```python
from build123d import *

# Parameters (mm, degrees)
SKETCH_W        = 32
SKETCH_H        = 20
PAD_DEPTH       = 22
CHAMFER_SIZE    = 5
SKETCH001_W     = 32
SKETCH001_H     = 15
POCKET_DEPTH    = 22
SKETCH002_W     = 32
SKETCH002_H     = 1
POCKET001_DEPTH = 2
SKETCH003_W     = 32
SKETCH003_H     = 3.1
POCKET002_DEPTH = 2
SKETCH004_W     = 2
SKETCH004_H     = 1
SKETCH004_H_2   = 3.1
POCKET003_DEPTH = 20
PAD001_DEPTH    = 2
POCKET004_DEPTH = 20
SKETCH007_W     = 1
SKETCH007_H     = 15
POCKET005_DEPTH = 0.5
CHAMFER001_SIZE = 2


with BuildPart() as part:
    # Sketch → Pad (new body)
    with BuildSketch(Plane.XY):
        with Locations((16, -10)):
            Rectangle(SKETCH_W, SKETCH_H)
    extrude(amount=PAD_DEPTH)

    # Chamfer
    chamfer_edges = [part.edges().sort_by_distance(p)[0] for p in [
        (0, -20, 11),
    ]]
    chamfer(chamfer_edges, length=CHAMFER_SIZE)

    # Sketch001 → Pocket (cut)
    with BuildSketch(Plane.XY.offset(22)):
        with Locations((16, -7.5)):
            Rectangle(SKETCH001_W, SKETCH001_H)
    extrude(amount=-POCKET_DEPTH, mode=Mode.SUBTRACT)

    # Sketch002 → Pocket001 (cut)
    with BuildSketch(Plane(origin=(0, 0, 0), x_dir=(1, 0, 0), z_dir=(0, 0, -1))):
        with Locations((16, 19.5)):
            Rectangle(SKETCH002_W, SKETCH002_H)
    extrude(amount=-POCKET001_DEPTH, mode=Mode.SUBTRACT)

    # Sketch003 → Pocket002 (cut)
    with BuildSketch(Plane(origin=(0, 0, 0), x_dir=(1, 0, 0), z_dir=(0, 0, -1))):
        with Locations((16, 16.55)):
            Rectangle(SKETCH003_W, SKETCH003_H)
    extrude(amount=-POCKET002_DEPTH, mode=Mode.SUBTRACT)

    # Sketch004 → Pocket003 (cut)
    with BuildSketch(Plane(origin=(0, 0, 2), x_dir=(1, 0, 0), z_dir=(0, 0, -1))):
        with Locations((31, 19.5)):
            Rectangle(SKETCH004_W, SKETCH004_H)
        with Locations((31, 16.55)):
            Rectangle(SKETCH004_W, SKETCH004_H_2)
    extrude(amount=-POCKET003_DEPTH, mode=Mode.SUBTRACT)

    # Sketch005 → Pad001 (new body)
    with BuildSketch(Plane(origin=(0, 0, 2), x_dir=(1, 0, 0), z_dir=(0, 0, -1))):
        Polygon((3.1, 18.1), (3, 18), (5.0281, 18.1), align=None)
    extrude(amount=PAD001_DEPTH)

    # Sketch006 → Pocket004 (cut)
    with BuildSketch(Plane(origin=(0, 0, 2), x_dir=(1, 0, 0), z_dir=(0, 0, -1))):
        Polygon((30, 15), (1, 15), (3.1, 17.1), (30, 17.1), align=None)
    extrude(amount=-POCKET004_DEPTH, mode=Mode.SUBTRACT)

    # Sketch007 → Pocket005 (cut)
    with BuildSketch(Plane.XZ.offset(20)):
        with Locations((11.5, 12)):
            Rectangle(SKETCH007_W, SKETCH007_H)
        with Locations((14.5, 12)):
            Rectangle(SKETCH007_W, SKETCH007_H)
        with Locations((17.5, 12)):
            Rectangle(SKETCH007_W, SKETCH007_H)
        with Locations((20.5, 12)):
            Rectangle(SKETCH007_W, SKETCH007_H)
        with Locations((23.5, 12)):
            Rectangle(SKETCH007_W, SKETCH007_H)
    extrude(amount=-POCKET005_DEPTH, mode=Mode.SUBTRACT)

    # Chamfer001
    chamfer001_edges = [part.edges().sort_by_distance(p)[0] for p in [
        (32, -18.55, 0),
    ]]
    chamfer(chamfer001_edges, length=CHAMFER001_SIZE)


solid = part.part
```
Check sheet for the modelled part. Datum: model origin and axes. Units: mm. A direction names the side the tool comes from. Coordinates: 2 decimals unless noted, no trailing zeros. Write each loop counter-clockwise with the first axis right and the second up, starting at its lowest first coordinate (ties: lowest second). Pieces come first, ordered by that corner, then holes. Notation, with made-up numbers: (-9, 32.25) - (25, 32.25) arc R18 cw to (25, 48.25) - close; hole circle Ø10 at (4, 67.25). An arc over 180 degrees is marked (long way). One line per question, with ' | ' between items.
Item 1: Access from +Z, -Z, +X, -X, +Y, -Y to the whole of each face (thin tool, end or side, straight path). Record for faces 5 (the face through (30, -17.6, 11.9)), 6 (the face through (31, -18.6, 1)), 7 (the face through (17.5, -19.5, 12.1)).
Determined:
face 5: +Z, -Z, +X, +Y | face 6: -Z, +X, +Y, -Y | face 7: -Y
Item 2: Gauge pin test, flat ends, axial feed: P1, Ø4, axis at x = 15.5, z = 5, coming from the +Y side; P2, Ø3, axis at y = -18.5, z = 14.5, coming from the -X side; P3, Ø3, axis at y = -17.5, z = 13, coming from the -X side. Record the tip position at first contact, or that the pin passes through.
Determined:
P1: stops at y = -17.1 | P2: stops at x = 2 | P3: stops at x = 1
Item 3: Mould release check, pull along Z, two halves, no side actions. Record for faces 1 (the face through (23.5, -19.5, 12.1)), 2 (the face through (16.8, -19.5, 2)), 3 (the face through (30, -19.5, 11.9)), 4 (the face through (14.5, -19.5, 12.1)): pulls with the +Z half, pulls with the -Z half, needs draft (parallel to the pull), parting line crosses it, or undercut.
Determined:
face 1: undercut | face 2: pulls with the -Z half | face 3: needs draft | face 4: undercut
Item 4: Sectioned sample at C-C on y = -15.85. Record the boundary of the cut face in (x, z).
Determined:
outline: (0.85, 2) - (1.85, 2) - (1.85, 22) - (0.85, 22) - close
Item 5: Sectioned sample at A-A on x = 16. Record the boundary of the cut face in (y, z).
Determined:
outline: (-20, 2) - (-19, 2) - (-19, 0) - (-18.1, 0) - (-18.1, 2) - (-17.1, 2) - (-17.1, 22) - (-20, 22) - close
Item 6: Thickness scan on line 1 (X direction, y = -19.65, z = 8.5); line 2 (X direction, y = -17, z = 4.25); line 3 (Y direction, x = 9.5, z = 2.25). Record the ranges inside material, lowest first. Write a range as [from, to].
Determined:
line 1: x = [4.65, 11], [12, 14], [15, 17], [18, 20], [21, 23], [24, 30] | line 2: x = [2, 3] | line 3: y = [-20, -17.1]
